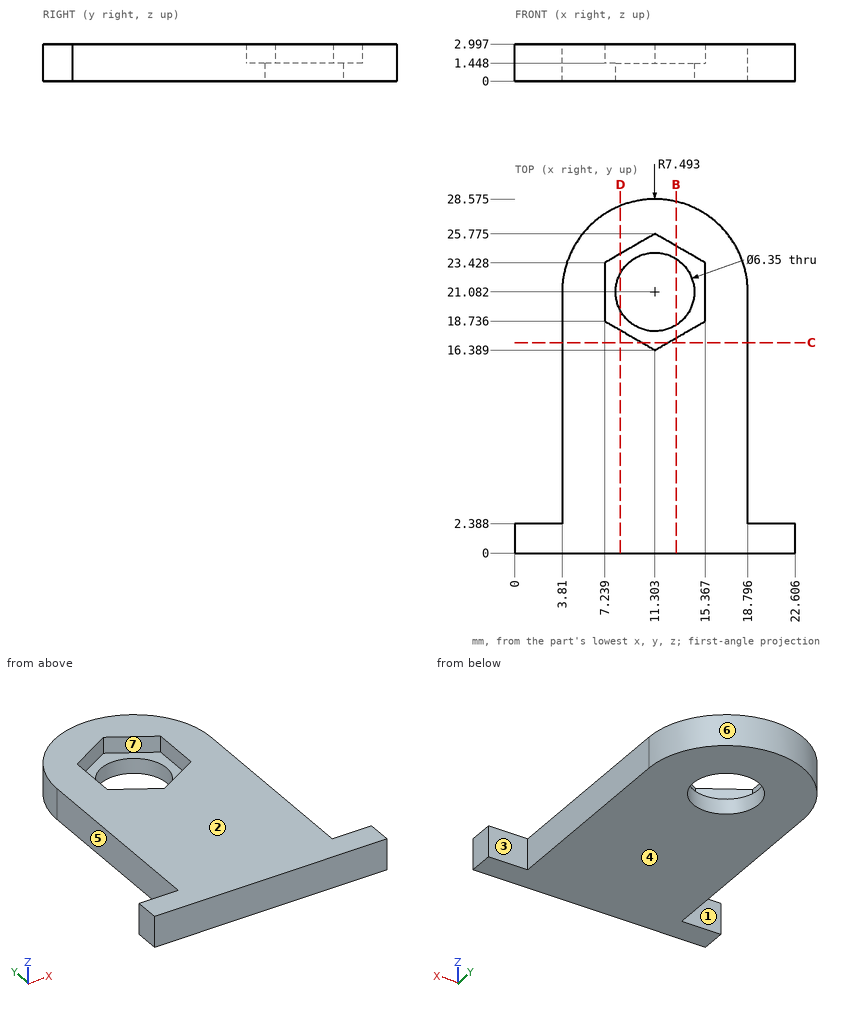
Verification items for this drawing (mm, ordinates from the low corner). A direction names the side the tool comes from. Give positions to 0.01 mm unless a question says otherwise; leave off trailing zeros. Order: outer loops, then holes, each group sorted by start corner. A loop starts at its lowest first (then second) coordinate and runs counter-clockwise, first axis right, second up.
1) Cross-section at C-C (y = 17). Record the boundary of the cut face in (x, z) (1 decimal).
Results are:
outline: (3.8, 0) - (18.8, 0) - (18.8, 3) - (12.4, 3) - (12.4, 1.4) - (10.2, 1.4) - (10.2, 3) - (3.8, 3) - close
2) Cross-section at D-D (x = 8.5). Record the boundary of the cut face in (y, z).
Results are:
outline: (0, 0) - (19.59, 0) - (19.59, 1.45) - (18.01, 1.45) - (18.01, 3) - (0, 3) - close; (22.57, 0) - (28.03, 0) - (28.03, 3) - (24.16, 3) - (24.16, 1.45) - (22.57, 1.45) - close
3) Draft check along X on the marked faces 4, 5, 6 and 7. Enter one of: released by +X, released by -X, zero draft, split by the parting line, or undercut.
Results are:
face 4: zero draft
face 5: released by -X
face 6: split by the parting line
face 7: undercut
4) Cross-section at B-B (x = 13). Record the boundary of the cut face in (y, z) (1 decimal).
Results are:
outline: (0, 0) - (18.4, 0) - (18.4, 1.4) - (17.4, 1.4) - (17.4, 3) - (0, 3) - close; (23.8, 0) - (28.4, 0) - (28.4, 3) - (24.8, 3) - (24.8, 1.4) - (23.8, 1.4) - close
5) Material ranges on probe 1 along Y at (x, z) = (20, 1.65); probe 2 along X at (y, z) = (9.5, 0.5); probe 3 along Y at (x, z) = (11.25, 1.05) (1 decimal), recorded low to high.
Results are:
probe 1: y = 0 to 2.39
probe 2: x = 3.81 to 18.8
probe 3: y = 0 to 17.9, 24.3 to 28.6
6) Gauge pin test, flat ends, axial feed: pin 1 (0.9 mm diameter, centred on x = 21, z = 2, fed in from +Y); pin 2 (1.7 mm diameter, centred on y = 20, z = 2, fed in from -X); pin 3 (1 mm diameter, centred on x = 16, z = 1, fed in from +Y). Record the tip position at first contact, or that the pin passes through.
Results are:
pin 1: stops at y = 2.39
pin 2: stops at x = 3.81
pin 3: stops at y = 27.29
7) Tool access check on the marked faces 1, 2 and 3. Record the directions out of +Z, -Z, +X, -X, +Y, -Y that give a thin tool (end or side, any length) a straight path to the whole face; none if there is none.
Results are:
face 1: +Z, -Z, -X, +Y
face 2: +Z, +X, -X, +Y, -Y
face 3: +Z, -Z, +X, +Y
